Autodesk Inventor part; units mm, degrees
ref_plane "YZ Plane" through (0, 0, 0) normal (1, 0, 0) x (0, 1, 0)
ref_plane "XZ Plane" through (0, 0, 0) normal (0, 1, 0) x (-1, 0, 0)
ref_plane "XY Plane" through (0, 0, 0) normal (0, 0, 1) x (1, 0, 0)
sketch "Эскиз1" plane through (0, 0, 0) normal (0, 1, 0) x (-1, 0, 0)
  line L0 (0, 0) -> (-92.3067, 154.5298)
  line L1 (-92.3067, 154.5298) -> (-92.3067, 214.5298)
  line L2 (-92.3067, 214.5298) -> (-0.3828, 306.4537)
  line L3 (-0.3828, 306.4537) -> (44.6172, 306.4537)
  line L4 (44.6172, 306.4537) -> (44.6172, 231.4537)
  line L5 (44.6172, 231.4537) -> (294.6172, 231.4537)
  line L6 (294.6172, 231.4537) -> (294.6172, 306.4537)
  line L7 (294.6172, 306.4537) -> (339.6172, 306.4537)
  line L8 (339.6172, 306.4537) -> (431.5411, 214.5298)
  line L9 (431.5411, 214.5298) -> (431.5411, 154.5298)
  line L10 (431.5411, 154.5298) -> (339.2344, 0)
  line L11 (339.2344, 0) -> (-0.7656, 0)
  point P0 (-92.3067, 184.5298)
  point P1 (431.5411, 184.5298)
  point P2 (-46.1534, 77.2649)
  point P3 (385.3877, 77.2649)
  point P4 (-46.3448, 260.4918)
  point P5 (385.5791, 260.4918)
  point P6 (294.6172, 268.9537)
  point P7 (44.6172, 268.9537)
  dimension "d0" = 180
  dimension "d1" = 130
  dimension "d2" = 45
  dimension "d3" = 75
  dimension "d4" = 60
  dimension "d5" = 180
  dimension "d6" = 250
  dimension "d7" = 340
extrude "Выдавливание1" add sketch "Эскиз1" along normal blind 100
sketch "Эскиз2" plane through (0, 100, 0) normal (0, 1, 0) x (1, 0, 0)
  point P0 (0, 0)
sketch "Эскиз3" plane through (92.3067, 0, 214.5298) normal (1, 0, 0) x (0, 0, -1)
  line L0 (33.7152, 148.0469) -> (238.2174, 0)
  line L1 (238.2174, 0) -> (332.909, 130.8007)
  line L2 (332.909, 130.8007) -> (135.9663, 223.0574)
  line L3 (135.9663, 223.0574) -> (33.7152, 148.0469)
  point P0 (214.5298, 0)
extrude "Выдавливание2" cut sketch "Эскиз3" against normal blind 600.5
sketch "Эскиз4" plane through (-407.5973, 100, 114.4458) normal (0, 0.81, -0.5864) x (1, 0, 0)
  line L0 (68.363, 141.2878) -> (407.5973, 141.2878)
  line L1 (407.5973, 141.2878) -> (475.9603, 0)
  line L2 (499.904, -32.4688) -> (475.9603, 0)
  line L3 (499.904, -81.0699) -> (499.904, -32.4688)
  line L4 (407.9801, -155.53) -> (499.904, -81.0699)
sketch "Эскиз5" plane through (0, 100, 0) normal (0, 1, 0) x (1, 0, 0)
  line L0 (-431.5411, -214.5298) -> (-339.6172, -306.4537)
  line L1 (-339.6172, -306.4537) -> (-294.6172, -306.4537)
  line L2 (-431.5411, -154.5298) -> (-431.5411, -214.5298)
  line L3 (-407.5973, -114.4458) -> (-431.5411, -154.5298)
  line L4 (-407.5973, -114.4458) -> (-339.2344, 0)
  line L5 (-339.2344, 0) -> (0, 0)
  line L6 (0, 0) -> (68.363, -114.4458)
  line L7 (92.3067, -154.5298) -> (68.363, -114.4458)
  line L8 (92.3067, -214.5298) -> (92.3067, -154.5298)
  line L9 (0.3828, -306.4537) -> (92.3067, -214.5298)
  line L10 (-44.6172, -306.4537) -> (0.3828, -306.4537)
  line L11 (-44.6172, -231.4537) -> (-44.6172, -306.4537)
  line L12 (-294.6172, -231.4537) -> (-44.6172, -231.4537)
  line L13 (-294.6172, -306.4537) -> (-294.6172, -231.4537)
  line L14 (0, -12.3836) -> (-332.2068, -12.3836)
  line L15 (-332.2068, -12.3836) -> (-396.966, -120.7964)
  line L16 (-396.966, -120.7964) -> (-419.1574, -157.9469)
  line L17 (-419.1574, -157.9469) -> (-419.1574, -209.4004)
  line L18 (-419.1574, -209.4004) -> (-334.4877, -294.0701)
  line L19 (-334.4877, -294.0701) -> (-307.0008, -294.0701)
  line L20 (-307.0008, -294.0701) -> (-307.0008, -219.0701)
  line L21 (-307.0008, -219.0701) -> (-32.2335, -219.0701)
  line L22 (-32.2335, -219.0701) -> (-32.2335, -294.0701)
  line L23 (-32.2335, -294.0701) -> (-4.7467, -294.0701)
  line L24 (-4.7467, -294.0701) -> (79.9231, -209.4004)
  line L25 (79.9231, -209.4004) -> (79.9231, -157.9469)
  line L26 (79.9231, -157.9469) -> (57.7316, -120.7964)
  line L27 (57.7316, -120.7964) -> (-10.6313, -6.3505)
  point P0 (-7.0275, -12.3836)
extrude "Выдавливание3" cut sketch "Эскиз5" against normal blind 93.75 contours L27 L26 L25 L24 L23 L22 L21 L20 L19 L18 L17 L16 L15 L14
sketch "Эскиз6" plane through (0, 6.25, 0) normal (0, 1, 0) x (1, 0, 0)
  line L0 (0, -241.7021) -> (50, -241.7021)
  line L1 (50, -241.7021) -> (50, -126.7021)
  line L2 (50, -126.7021) -> (0, -126.7021)
  line L3 (0, -126.7021) -> (0, -241.7021)
  line L4 (-334.4877, -294.0701) -> (-419.1574, -209.4004)
  line L5 (-386.9759, -241.5819) -> (-336.9759, -241.5819)
  line L6 (-336.9759, -241.5819) -> (-336.9759, -126.5819)
  line L7 (-336.9759, -126.5819) -> (-386.9759, -126.5819)
  line L8 (-386.9759, -126.5819) -> (-386.9759, -241.5819)
  point P0 (0, 0)
  point P1 (50, -184.2021)
  point P2 (0, -184.2021)
  point P3 (-336.9759, -184.0819)
  point P4 (-386.9759, -184.0819)
  point P5 (-361.9759, -241.5819)
  point P6 (-361.9759, -126.5819)
  point P7 (25, -241.7021)
  point P8 (25, -126.7021)
  dimension "d23" = 50
  dimension "d24" = 50
  dimension "d25" = 115
  dimension "d26" = 115
  dimension "d27" = 336.9759
extrude "Выдавливание4" cut sketch "Эскиз6" against normal blind 93.75
sketch "Эскиз7" plane through (-294.6172, 0, 306.4537) normal (1, 0, 0) x (0, 0, -1)
  line L0 (0, 100) -> (75, 100)
  line L1 (37.5, 100) -> (37.5, 0)
  line L2 (0, 0) -> (75, 0)
  line L3 (75, 0) -> (75, 100)
  line L4 (75, 50) -> (0, 50)
  line L5 (0, 0) -> (0, 100)
  circle A0 centre (37.5, 50) radius 15
  line L6 (-95.282, 50) -> (-21.0844, 50)
  line L7 (-58.1832, 95.9679) -> (-58.1832, 0)
  circle A1 centre (-58.1832, 47.9839) radius 15
  point P0 (306.4537, 0)
  dimension "d30" = 30
  dimension "d31" = 30
extrude "Выдавливание5" cut sketch "Эскиз7" against normal blind 20 contours A0 L4 L1 | L1 L4 A0 | L4 L1 A0 | L4 A0 L1 | A1 L7 L6 | L6 L7 A1 | L7 A1 L6 | L6 A1 L7
sketch "Эскиз8" plane through (-294.6172, 0, 231.4537) normal (0, 0, 1) x (1, 0, 0)
  point P0 (294.6172, 0)
sketch "Эскиз9" plane through (-44.6172, 0, 231.4537) normal (-1, 0, 0) x (0, 0, 1)
  line L0 (0, 0) -> (75, 0)
  line L1 (37.5, 0) -> (37.5, 100)
  line L2 (62.6164, 100) -> (-12.3836, 100)
  line L3 (75, 0) -> (75, 100)
  line L4 (75, 50) -> (1.0391, 50)
  line L5 (1.0391, 50) -> (0, 50)
  line L6 (0, 0) -> (0, 100)
  circle A0 centre (38.0196, 50) radius 15
  point P0 (-231.4537, 0)
  dimension "d34" = 30
extrude "Выдавливание6" cut sketch "Эскиз9" against normal blind 20 contours A0 L4 L1 | L1 L4 A0 | L4 A0 L1 | L1 A0 L4
properties part number "корпус"
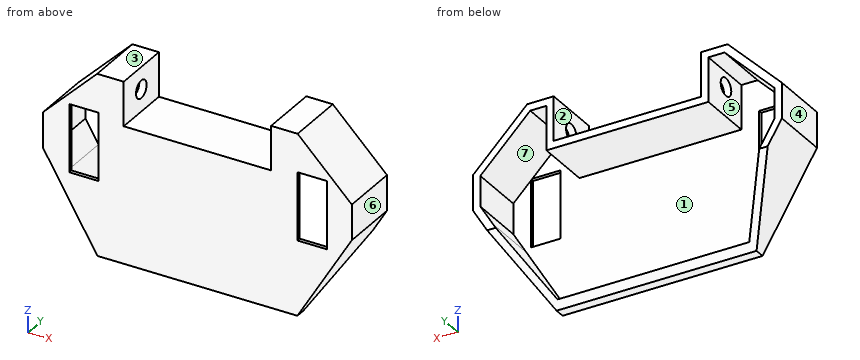
Part model, mm, in its own coordinate system. Face numbers are marked on the shaded views. A direction names the side the tool comes from. Give positions to 0.01 mm unless a question says otherwise; leave off trailing zeros. Write each loop counter-clockwise with the first axis right and the second up, starting at its lowest first coordinate (ties: lowest second). Pieces come first, ordered by that corner, then holes. Notation, with made-up numbers: (35, 30) -> (84, 30) arc R27 cw to (84, 46) -> close; hole circle Ø6 at (16.25, -31.5). An arc over 180 degrees is marked (long way). Put each result on its own line as item: value. Start each with the question number.
Item 1: Wall check: L1, parallel to Z at x = -303, y = 50; L2, parallel to X at y = 82, z = 177; L3, parallel to Z at x = -278.5, y = 14.5. Give the ranges that are in metal, low to high. Write a range as [from, to].
Item 2: Pin check, flat tips, straight feed: pin 1 Ø10 at (x, y) = (-67, 76) entering from +Z; pin 2 Ø2 at (x, z) = (-237, 132) entering from +Y; pin 3 Ø12 at (y, z) = (74.5, 249.5) entering from +X. Stop position of each tip, or through.
Item 3: Pull direction X, two halves, no side cores. Call the marked faces 4, 5, 6 and 7: pulls with the +X half, pulls with the -X half, needs draft (parallel to the pull), parting line crosses it, or undercut.
Item 4: Cut at D-D (x = 8). List the corners of the cut face in (y, z).
Item 5: Cut at C-C (y = 50). State how many separate pieces and enclosed holes the cut face has, then the cut area to 3 significant figures.
Item 6: Cut at A-A (z = 194). List the corners of the cut face in (x, y), then the cut area to 3 significant figures.
Item 7: Which spindle directions (+Z, -Z, +X, -X, +Y, -Y) get a long thin tool onto all of the face, cutting with end or side? Do the marked faces 1, 2 and 3. Say none if no direction does.
Item 8: Cut at B-B (x = -120.5). List the corners of the cut face in (y, z), then the cut area to 3 significant figures.
Answer list:
1. L1: z = [219.07, 253.95], [283.95, 306.45]
1. L2: x = [-431.54, -419.16], [79.92, 92.31]
1. L3: z = [0, 12.38], [219.07, 231.45]
2. pin 1: stops at z = 231.45
2. pin 2: stops at y = 6.25
2. pin 3: stops at x = 63.34
3. face 4: pulls with the -X half
3. face 5: undercut
3. face 6: pulls with the +X half
3. face 7: undercut
4. outline: (0, 13.39) -> (26.84, 13.39) -> (44.33, 37.54) -> (6.25, 37.54) -> (6.25, 126.7) -> (0, 126.7) -> close; (0, 241.7) -> (6.25, 241.7) -> (6.25, 281.32) -> (100, 281.32) -> (100, 298.84) -> (0, 298.84) -> close
5. separate pieces: 3
5. enclosed holes: 0
5. area: 12,900 mm2
6. outline: (-431.54, 0) -> (-386.98, 0) -> (-386.98, 6.25) -> (-419.16, 6.25) -> (-419.16, 100) -> (-431.54, 100) -> close; (-336.98, 0) -> (0, 0) -> (0, 6.25) -> (-336.98, 6.25) -> close; (50, 0) -> (92.31, 0) -> (92.31, 100) -> (79.92, 100) -> (79.92, 6.25) -> (50, 6.25) -> close
6. area: 4,970 mm2
7. face 1: +Y
7. face 2: +Z, +Y, -Y
7. face 3: +Z, +X, -X, +Y, -Y
8. outline: (0, 0) -> (17.15, 0) -> (26.11, 12.38) -> (6.25, 12.38) -> (6.25, 219.07) -> (100, 219.07) -> (100, 231.45) -> (0, 231.45) -> close
8. area: 2,800 mm2
